from build123d import *

# Parameters (mm, degrees)
SKETCH1_R                = 35
BOSS_EXTRUDE1_DEPTH      = 20
SKETCH2_R                = 25
CUT_EXTRUDE1_DEPTH       = 10
BOSS_EXTRUDE2_DEPTH      = 10
BOSS_EXTRUDE2_DEPTH_BACK = 10
SKETCH3_W                = 70
SKETCH3_H                = 40
BOSS_EXTRUDE3_DEPTH      = 20
BOSS_EXTRUDE3_DEPTH_BACK = 20
SKETCH5_R                = 3.5
CUT_EXTRUDE2_START       = 27
SKETCH6_R                = 25
CUT_EXTRUDE2_DEPTH       = 27


with BuildPart() as part:
    # Sketch1 → Boss-Extrude1 (new body)
    with BuildSketch(Plane(origin=(0, 0, 0), x_dir=(0, 0, -1), z_dir=(1, 0, 0))):
        Circle(SKETCH1_R)
    extrude(amount=BOSS_EXTRUDE1_DEPTH)

    # Sketch2 → Cut-Extrude1 (cut)
    with BuildSketch(Plane(origin=(0, 0, 0), x_dir=(0, 0, -1), z_dir=(1, 0, 0))):
        Circle(SKETCH2_R)
    extrude(amount=CUT_EXTRUDE1_DEPTH, mode=Mode.SUBTRACT)

    # Sketch3 → Boss-Extrude2 (add, two sides: drawn at the far end of the back side and taken through both)
    with BuildSketch(Plane(origin=(0, 0, 0), x_dir=(1, 0, 0), z_dir=(0, 1, 0)).offset(-BOSS_EXTRUDE2_DEPTH_BACK)):
        with Locations((35.208452682, 0)):
            Rectangle(SKETCH3_W, SKETCH3_H)
    extrude(amount=BOSS_EXTRUDE2_DEPTH + BOSS_EXTRUDE2_DEPTH_BACK)

    # Sketch5 → Boss-Extrude3 (add, two sides: drawn at the far end of the back side and taken through both)
    with BuildSketch(Plane(origin=(0, 0, 0), x_dir=(1, 0, 0), z_dir=(0, 1, 0)).offset(-BOSS_EXTRUDE3_DEPTH_BACK)):
        with Locations(Location((40, -10, 0), (0, 0, 270))):
            Circle(SKETCH5_R)
        with Locations(Location((40, 10, 0), (0, 0, 270))):
            Circle(SKETCH5_R)
        with Locations(Location((60, 10, 0), (0, 0, 270))):
            Circle(SKETCH5_R)
        with Locations(Location((60, -10, 0), (0, 0, 270))):
            Circle(SKETCH5_R)
    extrude(amount=BOSS_EXTRUDE3_DEPTH + BOSS_EXTRUDE3_DEPTH_BACK)

    # Sketch6 → Cut-Extrude2 (cut)
    with BuildSketch(Plane.ZY.offset(-10).offset(CUT_EXTRUDE2_START)):
        with Locations(Location((0, 0, 0), (0, 0, 180))):
            Circle(SKETCH6_R)
    extrude(amount=-CUT_EXTRUDE2_DEPTH, mode=Mode.SUBTRACT)


solid = part.part
Geometry: final body of the model. Coordinates: model frame, mm. A direction names the side the tool comes from. Coordinates: 2 decimals unless noted, no trailing zeros. Order: outer loops, then holes, each group sorted by start corner. A loop starts at its lowest first (then second) coordinate and runs counter-clockwise, first axis right, second up.
(1) Draft query along X for faces 5 (the face through (57.9, -15.1, -12.8)), 6 (the face through (10, 0, 0)), 7 (the face through (60, 20, 10)). Return one class per face: pulls with the +X half, pulls with the -X half, needs draft (parallel to the pull), parting line crosses it, or undercut.
(2) Section query B-B (y = -17). Return the cut outline in (x, z), plus the area to 3 significant figures.
(3) Material intervals for probe 1 along Y at (x, z) = (6, 0); probe 2 along Y at (x, z) = (48, 0); probe 3 along X at (y, z) = (-23, -10.5), sorted ascending.
(4) First-contact query: pin 1 (7.5 mm diameter, centred on x = 40, z = -11, fed in from -Y); pin 2 (1.5 mm diameter, centred on x = 49.5, y = 1.5, fed in from -Z); pin 3 (1.5 mm diameter, centred on y = 19, z = 0.5, fed in from +X); pin 4 (4 mm diameter, centred on y = 8, z = 26.5, fed in from -X). Flat tips, straight axial feed; report the tip coordinate or a pass-through.
(5) Section query C-C (z = 0). Return the cut outline in (x, y), plus the area to 3 significant figures.
(6) Section query D-D (x = 6.5). Return the cut outline in (y, z), plus the area to 3 significant figures.
(7) Section query A-A (x = 60). Return the cut outline in (y, z).
(8) Access query for faces 1 (the face through (60, -20, -10)), 2 (the face through (60.154, -15.07, 6.503)), 3 (the face through (60, 20, -10)), 4 (the face through (45, 0, 20)). Directions: +Z, -Z, +X, -X, +Y, -Y. A direction counts if a zero-diameter tool reaches every point of the face in a straight line with its end or side. Return the directions, or none.
Solution:
1. face 5: undercut
1. face 6: pulls with the -X half
1. face 7: needs draft
2. outline: (0, -30.59) - (20, -30.59) - (20, 30.59) - (0, 30.59) - (0, 18.33) - (10, 18.33) - (10, -18.33) - (0, -18.33) - close; circle Ø7 at (40, -10); circle Ø7 at (40, 10); circle Ø7 at (60, -10); circle Ø7 at (60, 10)
2. area: 1,010 mm2
3. probe 1: y = -35 to -25, 25 to 35
3. probe 2: y = -10 to 10
3. probe 3: x = 0 to 20
4. pin 1: stops at y = -20
4. pin 2: stops at z = -20
4. pin 3: stops at x = 20
4. pin 4: stops at x = 0
5. outline: (0, -35) - (20, -35) - (20, -10) - (70.21, -10) - (70.21, 10) - (20, 10) - (20, 35) - (0, 35) - (0, 25) - (10, 25) - (10, -25) - (0, -25) - close
5. area: 1,900 mm2
6. outline: circle Ø70 at (0, 0); hole circle Ø50 at (0, 0)
6. area: 1,880 mm2
7. outline: (-20, -13.5) - (-10, -13.5) - (-10, -20) - (10, -20) - (10, -13.5) - (20, -13.5) - (20, -6.5) - (10, -6.5) - (10, 6.5) - (20, 6.5) - (20, 13.5) - (10, 13.5) - (10, 20) - (-10, 20) - (-10, 13.5) - (-20, 13.5) - (-20, 6.5) - (-10, 6.5) - (-10, -6.5) - (-20, -6.5) - close
8. face 1: +Z, -Z, +X, -Y
8. face 2: -Y
8. face 3: +Z, -Z, +X, +Y
8. face 4: +Z, +X, +Y, -Y
